Part model, mm, in its own coordinate system. A direction names the side the tool comes from. Round coordinates to 2 decimals unless told otherwise and drop trailing zeros. Write each loop counter-clockwise with the first axis right and the second up, starting at its lowest first coordinate (ties: lowest second). Pieces come first, ordered by that corner, then holes. Notation, with made-up numbers: M 78,58.25 L 110,58.25 A15 ccw 110,73.25 Z; hole C 15,14.25 d9. An arc over 180 degrees is marked long. Use a Markdown table: item, result. Add a question column.
1) Which spindle directions (+Z, -Z, +X, -X, +Y, -Y) get a long thin tool onto all of the face, cutting with end or side? Do faces 5 (the face through (0, 21, 5.5)), 6 (the face through (-10.43, 39.17, -4.9)). Say none if no direction does.
2) Slice it at D-D on x = 5.25. Write the cut outline in (y, z), plus the area to 3 significant figures.
3) Two-plate mould, pull along Z, no slides. Class faces 1 (the face through (0, 5.75, 0)), 2 (the face through (-10.43, 2.92, -4.9)), 3 (the face through (0, 21, 11.5)), 4 (the face through (-7, 39, 0)): released by +Z, released by -Z, zero draft, split by the parting line, or undercut.
4) Slice it at A-A on z = 5. Write the cut outline in (x, y).
5) Slice it at C-C on z = 0. Write the cut outline in (x, y), plus the area to 4 significant figures.
6) Drop flat-ended pins along their axis: P1, Ø10, axis at x = -1, y = 26.5, coming from the -Z side; P2, Ø10, axis at y = 28.5, z = -3, coming from the -X side. Give the stop position or say it passes through.
7) Slice it at B-B on y = 37. Write the cut outline in (x, z).
8) Wall check: probe 1 along X at (y, z) = (40.45, 0); probe 2 along Y at (x, z) = (4.75, -3.5); probe 3 along Z at (x, y) = (-5.25, 38). Give the ranges that are in metal, low to high.
```python
from build123d import *

# Parameters (mm, degrees)
SKETCH1_W           = 22
SKETCH1_H           = 6
SKETCH1_H_2         = 11
SKETCH1_R           = 1.75
BOSS_EXTRUDE1_DEPTH = 42
SKETCH2_W           = 22
SKETCH2_H           = 30.5
CUT_EXTRUDE1_DEPTH  = 11
FILLET1_R           = 2


with BuildPart() as part:
    # Sketch1 → Boss-Extrude1 (new body)
    with BuildSketch(Plane(origin=(0, 0, 0), x_dir=(1, 0, 0), z_dir=(0, 1, 0))):
        with Locations((0, -8.5)):
            Rectangle(SKETCH1_W, SKETCH1_H)
        Rectangle(SKETCH1_W, SKETCH1_H_2)
        with Locations((5.25, 0)):
            Circle(SKETCH1_R, mode=Mode.SUBTRACT)
        with Locations((-5.25, 0)):
            Circle(SKETCH1_R, mode=Mode.SUBTRACT)
    extrude(amount=BOSS_EXTRUDE1_DEPTH)

    # Sketch2 → Cut-Extrude1 (cut)
    with BuildSketch(Plane(origin=(0, 0, -5.5), x_dir=(-1, 0, 0), z_dir=(0, 0, -1))):
        with Locations((0, 21)):
            Rectangle(SKETCH2_W, SKETCH2_H)
    extrude(amount=-CUT_EXTRUDE1_DEPTH, mode=Mode.SUBTRACT)

    # Fillet1
    fillet1_edges = [part.edges().sort_by_distance(p)[0] for p in [
        (0, 0, 11.5),
        (-11, 39.125, -5.5),
        (11, 39.125, -5.5),
        (-11, 2.875, -5.5),
        (11, 2.875, -5.5),
        (0, 42, 11.5),
    ]]
    fillet(fillet1_edges, radius=FILLET1_R)


solid = part.part
```
Entries:
| question | item | result |
|---|---|---|
| 1 | face 5 | -Z, +X, -X |
| 1 | face 6 | -Z, -X, +Y, -Y |
| 2 | outline | M 0,-5.5 L 5.75,-5.5 L 5.75,-1.75 L 0,-1.75 Z; M 0,1.75 L 5.75,1.75 L 5.75,5.5 L 36.25,5.5 L 36.25,1.75 L 42,1.75 L 42,9.5 A2 ccw 40,11.5 L 2,11.5 A2 ccw 0,9.5 Z; M 36.25,-5.5 L 42,-5.5 L 42,-1.75 L 36.25,-1.75 Z |
| 2 | area | 337 mm^2 |
| 3 | face 1 | zero draft |
| 3 | face 2 | released by -Z |
| 3 | face 3 | released by +Z |
| 3 | face 4 | undercut |
| 4 | outline | M -11,0 L 11,0 L 11,5.75 L -11,5.75 Z; M -11,36.25 L 11,36.25 L 11,42 L -11,42 Z |
| 5 | outline | M -11,0 L -7,0 L -7,5.75 L -11,5.75 Z; M -11,36.25 L -7,36.25 L -7,42 L -11,42 Z; M -3.5,0 L 3.5,0 L 3.5,5.75 L -3.5,5.75 Z; M -3.5,36.25 L 3.5,36.25 L 3.5,42 L -3.5,42 Z; M 7,0 L 11,0 L 11,5.75 L 7,5.75 Z; M 7,36.25 L 11,36.25 L 11,42 L 7,42 Z |
| 5 | area | 172.5 mm^2 |
| 6 | P1 | stops at z = 5.5 |
| 6 | P2 | passes through |
| 7 | outline | M -11,-3.5 A2 ccw -9,-5.5 L 9,-5.5 A2 ccw 11,-3.5 L 11,11.5 L -11,11.5 Z; hole C -5.25,0 d3.5; hole C 5.25,0 d3.5 |
| 8 | probe 1 | x = -11 to -7, -3.5 to 3.5, 7 to 11 |
| 8 | probe 2 | y = 0 to 5.75, 36.25 to 42 |
| 8 | probe 3 | z = -5.5 to -1.75, 1.75 to 11.5 |
